from build123d import *

# Parameters (mm, degrees)
CYLINDER013_R     = 15
CYLINDER013_DEPTH = 7
CYLINDER012_R     = 21
CYLINDER012_DEPTH = 7


with BuildPart() as bearing_inner:
    # Cylinder013 → Cylinder013 (new body)
    with BuildSketch(Plane.XY):
        Circle(CYLINDER013_R)
    extrude(amount=CYLINDER013_DEPTH)


with BuildPart() as bearing:
    # Cylinder012 → Cylinder012 (new body)
    with BuildSketch(Plane.XY):
        Circle(CYLINDER012_R)
    extrude(amount=CYLINDER012_DEPTH)

    # Cut001: cut bearing inner
    add(bearing_inner.part, mode=Mode.SUBTRACT)


with BuildPart() as bearing_1:
    # Cut001 placement: moved
    add(bearing.part.moved(Location((0, 0, 16.5))))


solid = bearing_1.part
Here's how the part is built. I have some questions about the finished solid (model axes, mm). Give positions to 0.01 mm unless a question says otherwise; leave off trailing zeros. Order: outer loops, then holes, each group sorted by start corner. A loop starts at its lowest first (then second) coordinate and runs counter-clockwise, first axis right, second up. Notation, with made-up numbers: M -39,61 L -10,61 A29 ccw -10,88 Z; hole C 53,-8 d2. An arc over 180 degrees is marked long. Answer as a JSON object with one key per item and string values. Group by question number.
1) We'd pull the mould along Y, two halves only. Please class faces 1 (the cylindrical face through (20.03, 6.31, 19.95)), 2 (the cylindrical face through (-14.985, 0.66, 19.951)), 3 (the flat face through (9, -14, 16.5)): pulls with the +Y half, pulls with the -Y half, needs draft (parallel to the pull), parting line crosses it, or undercut.
2) I'm going to push flat-ended pins straight in: pin 1 Ø1 at (x, z) = (-8, 22) entering from +Y; pin 2 Ø24 at (x, y) = (0, 0) entering from -Z; pin 3 Ø1.5 at (x, z) = (-15, 21) entering from +Y. Where does each tip first touch, or does it pass through?
3) Suppose I cut it at A-A, the plane x = 0. Write out the boundary of the cut face in (y, z).
4) Suppose I cut it at C-C, the plane z = 17.5. Write out the boundary of the cut face in (x, y).
5) Please list where these lines run through material, in increasing order: L1, parallel to X at y = -0.5, z = 20.5; L2, parallel to Y at x = 0, z = 22; L3, parallel to X at y = 13, z = 21.5. Write a range as [from, to].
6) Suppose I cut it at D-D, the plane x = -17. Write out the boundary of the cut face in (y, z).
Results found:
{
 "1": {"face 1": "parting line crosses it", "face 2": "undercut", "face 3": "needs draft"},
 "2": {"pin 1": "y = 19.62", "pin 2": "through", "pin 3": "y = 15.43"},
 "3": {"outline": "M -21,16.5 L -15,16.5 L -15,23.5 L -21,23.5 Z; M 15,16.5 L 21,16.5 L 21,23.5 L 15,23.5 Z"},
 "4": {"outline": "C 0,0 d42; hole C 0,0 d30"},
 "5": {"L1": "[-20.99, -14.99], [14.99, 20.99]", "L2": "[-21, -15], [15, 21]", "L3": "[-16.49, -7.48], [7.48, 16.49]"},
 "6": {"outline": "M -12.33,16.5 L 12.33,16.5 L 12.33,23.5 L -12.33,23.5 Z"}
}
